Geometry check sheet. Reference: the model listing, model coordinates, mm. Face numbers are marked on the shaded views. A direction names the side the tool comes from. Round coordinates to 2 decimals unless told otherwise and drop trailing zeros. Write each loop counter-clockwise with the first axis right and the second up, starting at its lowest first coordinate (ties: lowest second). Pieces come first, ordered by that corner, then holes. Notation, with made-up numbers: (0.5, -13.5) -> (38.5, -13.5) arc R21 cw to (38.5, 7.5) -> close; hole circle Ø5 at (81.25, 47.25). An arc over 180 degrees is marked (long way). Use a Markdown table: item, result.
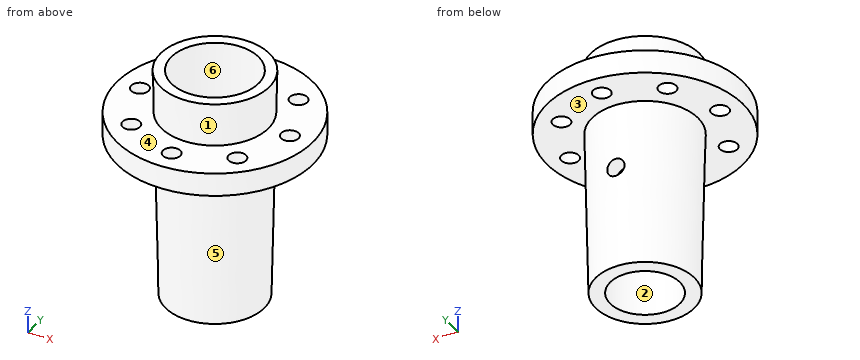
```python
from build123d import *

# Parameters (mm, degrees)
SCHIZZO5_W                  = 15
SCHIZZO5_H                  = 30
SCHIZZO7_R                  = 3
TAGLIO_ESTRUSIONE1_DEPTH    = 24
RIPETIZIONECIRCOLARE1_COUNT = 8
SCHIZZO8_R                  = 3
TAGLIO_ESTRUSIONE2_DEPTH    = 34.75


with BuildPart() as part:
    # Schizzo3 → Rivoluzione2 (revolve)
    with BuildSketch(Plane(origin=(0, 0, 0), x_dir=(1, 0, 0), z_dir=(0, 1, 0))):
        Polygon((-17, 40), (-12, 40), (-12, -40), (-18.75, -40), (-18.421875, -25), (-33.75, -25), (-33.75, -17), (-18.246875, -17), align=None)
    revolve(axis=Axis((0, 0, -65.081098712), (0, 0, 1)))

    # Schizzo5 → Taglia-Rivoluzione1 (revolve, cut)
    with BuildSketch(Plane(origin=(0, 0, 0), x_dir=(1, 0, 0), z_dir=(0, 1, 0))):
        with Locations((-7.5, -25)):
            Rectangle(SCHIZZO5_W, SCHIZZO5_H)
    revolve(axis=Axis((0, 0, -67.558392607), (0, 0, 1)), mode=Mode.SUBTRACT)

    # Schizzo7 → Taglio-Estrusione1 (cut, through all)
    with BuildSketch(Plane(origin=(0, 0, 17), x_dir=(-1, 0, 0), z_dir=(0, 0, -1))):
        with Locations((0, -26)):
            Circle(SCHIZZO7_R)
    taglio_estrusione1 = extrude(amount=-TAGLIO_ESTRUSIONE1_DEPTH, mode=Mode.SUBTRACT)

    # RipetizioneCircolare1: Taglio-Estrusione1 ×8 about axis
    ripetizionecircolare1_axis = Axis((0, 0, 0), (0, 0, 1))
    for i in range(1, RIPETIZIONECIRCOLARE1_COUNT):
        add(taglio_estrusione1.rotate(ripetizionecircolare1_axis, i * 360 / RIPETIZIONECIRCOLARE1_COUNT), mode=Mode.SUBTRACT)

    # Schizzo8 → Taglio-Estrusione2 (cut, through all)
    with BuildSketch(Plane(origin=(0, 0, 0), x_dir=(1, 0, 0), z_dir=(0, 1, 0))):
        with Locations((0, 5)):
            Circle(SCHIZZO8_R)
    extrude(amount=TAGLIO_ESTRUSIONE2_DEPTH, mode=Mode.SUBTRACT)


solid = part.part
```
(1) Section check B-B on y = 0. Record the cut outline in (x, z).
A:
| item | result |
|---|---|
| outline | (-33.75, 17) -> (-29, 17) -> (-29, 25) -> (-33.75, 25) -> close; (-23, 17) -> (-18.25, 17) -> (-17, -40) -> (-12, -40) -> (-12, 10) -> (-15, 10) -> (-15, 40) -> (-18.75, 40) -> (-18.42, 25) -> (-23, 25) -> close; (12, -40) -> (17, -40) -> (18.25, 17) -> (23, 17) -> (23, 25) -> (18.42, 25) -> (18.75, 40) -> (15, 40) -> (15, 10) -> (12, 10) -> close; (29, 17) -> (33.75, 17) -> (33.75, 25) -> (29, 25) -> close |
(2) Section check D-D on x = 0. State how many separate pieces and enclosed holes the cut face has, plus the area to 3 significant figures.
A:
| item | result |
|---|---|
| separate pieces | 5 |
| enclosed holes | 0 |
| area | 876 mm2 |
(3) Access from +Z, -Z, +X, -X, +Y, -Y to the whole of each face (thin tool, end or side, straight path). Record for the marked faces 1, 2 and 3.
A:
| item | result |
|---|---|
| face 1 | none |
| face 2 | +Z, -Z |
| face 3 | -Z |
(4) Gauge pin test, flat ends, axial feed: pin 1 Ø5.5 at (x, y) = (26, 0) entering from +Z; pin 2 Ø12 at (y, z) = (10, -16) entering from -X; pin 3 Ø10 at (x, y) = (-25.5, 9.5) entering from +Z; pin 4 Ø1 at (y, z) = (-10.5, 1.5) entering from -X. Record the tip position at first contact, or that the pin passes through.
A:
| item | result |
|---|---|
| pin 1 | passes through |
| pin 2 | stops at x = -17.07 |
| pin 3 | stops at z = 25 |
| pin 4 | stops at x = -14.86 |
(5) Thickness scan on line 1 (X direction, y = 0, z = 23.5); line 2 (Y direction, x = 20, z = 18). Record the ranges inside material, lowest first.
A:
| item | result |
|---|---|
| line 1 | x = -33.75 to -29, -23 to -15, 15 to 23, 29 to 33.75 |
| line 2 | y = -27.19 to -20.91, -15.86 to 15.86, 20.91 to 27.19 |
(6) Section check A-A on y = 26. Record the cut outline in (x, z).
A:
| item | result |
|---|---|
| outline | (-21.52, 17) -> (-3, 17) -> (-3, 25) -> (-21.52, 25) -> close; (3, 17) -> (21.52, 17) -> (21.52, 25) -> (3, 25) -> close |
(7) Release check for a two-part mould opening along X. For the marked faces 4, 5 and 6 record: +X half, -X half, draft (parallel to the pull), parting line (faces both ways), or undercut.
A:
| item | result |
|---|---|
| face 4 | draft |
| face 5 | parting line |
| face 6 | undercut |
